Can you work these out from the drawing? Everything is in mm from the part's minimum corner. A direction names the side the tool comes from. Round coordinates to 2 decimals unless told otherwise and drop trailing zeros. Order: outer loops, then holes, each group sorted by start corner. A loop starts at its lowest first (then second) coordinate and runs counter-clockwise, first axis right, second up. Notation, with made-up numbers: (26.25, 85.25) -> (75.25, 85.25) arc R20 ccw to (75.25, 102.25) -> close; hole circle Ø3 at (10.5, -0.75). An arc over 180 degrees is marked (long way). One line per item, written item: value.
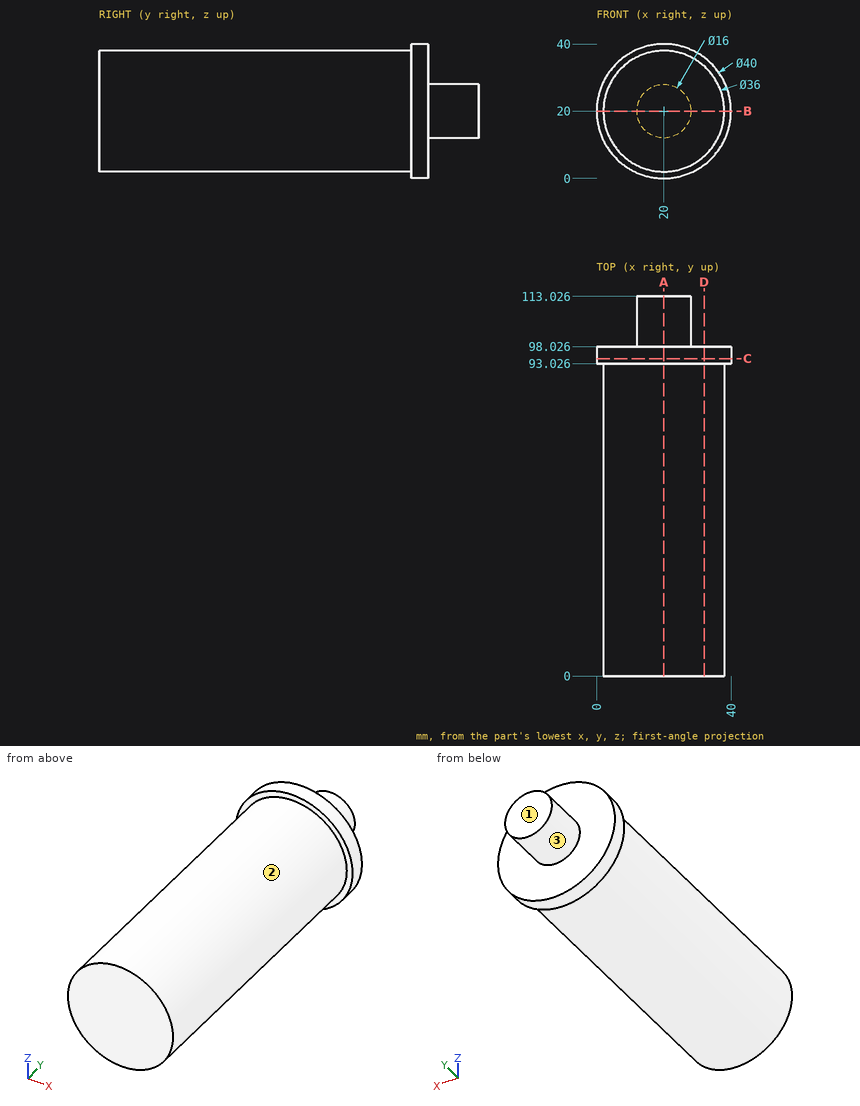
Q1. For P1, Ø6, axis at x = 22.5, y = 68.5, coming from the +Z side; P2, Ø10, axis at y = 32.5, z = 29, coming from the +X side; P3, Ø1, axis at x = 7.5, z = 8.5, coming from the +Y side, each with a flat end and sliding along its axis, tell me the tip position at first contact or that it passes through.
Answers:
P1: z = 38
P2: x = 37.55
P3: y = 98.03
Q2. I want a section at B-B on z = 20. Write out the boundary of the cut face in (x, y).
Answers:
outline: (0, 93.03) -> (2, 93.03) -> (2, 0) -> (38, 0) -> (38, 93.03) -> (40, 93.03) -> (40, 98.03) -> (28, 98.03) -> (28, 113.03) -> (12, 113.03) -> (12, 98.03) -> (0, 98.03) -> close
Q3. I want a section at C-C on y = 94.5. Write out the boundary of the cut face in (x, z), then the cut area to 3 significant figures.
Answers:
outline: circle Ø40 at (20, 20)
area: 1,260 mm2
Q4. I want a section at D-D on x = 32. Write out the boundary of the cut face in (y, z).
Answers:
outline: (0, 6.58) -> (93.03, 6.58) -> (93.03, 4) -> (98.03, 4) -> (98.03, 36) -> (93.03, 36) -> (93.03, 33.42) -> (0, 33.42) -> close
Q5. I need wall thicknesses on line 1 along Y through (x, z) = (10.5, 37); line 2 along Y through (x, z) = (11.5, 26.5); line 3 along Z through (x, y) = (36.5, 95.5) (1 decimal). Which ranges of each line are inside material? Lowest first, please.
Answers:
line 1: 93.03 to 98.03
line 2: 0 to 98.03
line 3: 8.7 to 31.3
Q6. Which directions (+Z, -Z, +X, -X, +Y, -Y) give clear straight access to the entire face, cutting with the end or side of a thin tool? Please do the marked faces 1, 2 and 3.
Answers:
face 1: +Z, -Z, +X, -X, +Y
face 2: -Y
face 3: +Y
Q7. I want a section at A-A on x = 20. Write out the boundary of the cut face in (y, z).
Answers:
outline: (0, 2) -> (93.03, 2) -> (93.03, 0) -> (98.03, 0) -> (98.03, 12) -> (113.03, 12) -> (113.03, 28) -> (98.03, 28) -> (98.03, 40) -> (93.03, 40) -> (93.03, 38) -> (0, 38) -> close
